Read the model definition and answer for the solid it produces. Units are mm, in the model's axes. Face numbers are marked on the shaded views. A direction names the side the tool comes from. Coordinates: 2 decimals unless noted, no trailing zeros. Loops run counter-clockwise (first coordinate to the right, second up) from the corner with the lowest first, then second, coordinate; pieces in that order, holes last. Notation, with made-up numbers: (5.5, -33.75) -> (25.5, -33.75) arc R14 ccw to (25.5, -25.75) -> close; hole circle Ø2 at (-34.5, 12). An arc over 180 degrees is marked (long way). One line per question, with ' | ' between items. Start each with the question number.
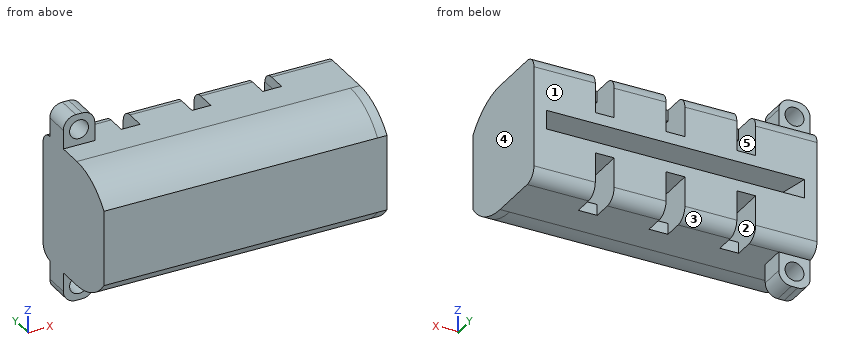
```python
from build123d import *

# Parameters (mm, degrees)
SKETCH1_W            = 90
SKETCH1_H            = 20
BOSS_EXTRUDE1_DEPTH  = 20
SKETCH2_W            = 90
SKETCH2_H            = 3
CUT_EXTRUDE1_DEPTH   = 10
SKETCH3_W            = 3
SKETCH3_H            = 5
CUT_EXTRUDE2_DEPTH   = 10
SKETCH4_W            = 3
SKETCH4_H            = 1.75
SKETCH4_W_2          = 2.997618753
SKETCH4_W_3          = 3.002941468
CUT_EXTRUDE3_DEPTH   = 5
SKETCH5_W            = 1.5
SKETCH5_H            = 3
BOSS_EXTRUDE2_DEPTH  = 10
SKETCH6_W            = 1.5
SKETCH6_H            = 3
BOSS_EXTRUDE3_DEPTH  = 18
BOSS_EXTRUDE4_DEPTH  = 5
FILLET1_START        = 8.5
FILLET1_DEPTH        = 3
FILLET1_START_2      = 8
FILLET1_2_DEPTH      = 4
FILLET2_R            = 10
SKETCH8_W            = 20.140972823
SKETCH8_H            = 2
CUT_EXTRUDE4_DEPTH   = 119
FILLET3_R            = 2
SKETCH9_W            = 5
SKETCH9_H            = 4
BOSS_EXTRUDE6_DEPTH  = 5
SKETCH11_W           = 5
SKETCH11_H           = 4
BOSS_EXTRUDE7_DEPTH  = 5
SKETCH12_R           = 1.5
CUT_EXTRUDE5_DEPTH   = 24
FILLET4_R            = 2
SKETCH14_W           = 71.95999564
SKETCH14_H           = 44.647918029
CUT_EXTRUDE8_DEPTH   = 55
BOSS_EXTRUDE8_START  = 1.5
BOSS_EXTRUDE8_DEPTH  = 1.5
SKETCH16_W           = 5.976122604
SKETCH16_H           = 3
CUT_EXTRUDE9_DEPTH   = 10
SKETCH17_W           = 2
SKETCH17_H           = 3
BOSS_EXTRUDE9_DEPTH  = 10
BOSS_EXTRUDE10_DEPTH = 5


with BuildPart() as part:
    # Sketch1 → Boss-Extrude1 (new body)
    with BuildSketch(Plane.XY):
        with Locations((45, -10)):
            Rectangle(SKETCH1_W, SKETCH1_H)
    extrude(amount=BOSS_EXTRUDE1_DEPTH)

    # Sketch2 → Cut-Extrude1 (cut)
    with BuildSketch(Plane(origin=(0, 0, 0), x_dir=(1, 0, 0), z_dir=(0, 1, 0))):
        with Locations((45, -10)):
            Rectangle(SKETCH2_W, SKETCH2_H)
    extrude(amount=-CUT_EXTRUDE1_DEPTH, mode=Mode.SUBTRACT)

    # Sketch3 → Cut-Extrude2 (cut)
    with BuildSketch(Plane(origin=(0, 0, 0), x_dir=(1, 0, 0), z_dir=(0, 1, 0))):
        with Locations((11.25, -15.75)):
            Rectangle(SKETCH3_W, SKETCH3_H)
        with Locations((22.5, -15.75)):
            Rectangle(SKETCH3_W, SKETCH3_H)
        with Locations((33.75, -15.75)):
            Rectangle(SKETCH3_W, SKETCH3_H)
        with Locations((45, -15.75)):
            Rectangle(SKETCH3_W, SKETCH3_H)
        with Locations((56.25, -15.75)):
            Rectangle(SKETCH3_W, SKETCH3_H)
        with Locations((67.5, -15.75)):
            Rectangle(SKETCH3_W, SKETCH3_H)
        with Locations((78.75, -15.75)):
            Rectangle(SKETCH3_W, SKETCH3_H)
        with Locations((11.25, -4.25)):
            Rectangle(SKETCH3_W, SKETCH3_H)
        with Locations((22.5, -4.25)):
            Rectangle(SKETCH3_W, SKETCH3_H)
        with Locations((33.75, -4.25)):
            Rectangle(SKETCH3_W, SKETCH3_H)
        with Locations((45, -4.25)):
            Rectangle(SKETCH3_W, SKETCH3_H)
        with Locations((56.25, -4.25)):
            Rectangle(SKETCH3_W, SKETCH3_H)
        with Locations((67.5, -4.25)):
            Rectangle(SKETCH3_W, SKETCH3_H)
        with Locations((78.75, -4.25)):
            Rectangle(SKETCH3_W, SKETCH3_H)
    extrude(amount=-CUT_EXTRUDE2_DEPTH, mode=Mode.SUBTRACT)

    # Sketch4 → Cut-Extrude3 (cut)
    with BuildSketch(Plane(origin=(0, 0, 0), x_dir=(1, 0, 0), z_dir=(0, 1, 0))):
        with Locations((56.25, -19.125)):
            Rectangle(SKETCH4_W, SKETCH4_H)
        with Locations((67.5, -19.125)):
            Rectangle(SKETCH4_W, SKETCH4_H)
        Polygon((77.25, -18.25), (77.25, -20), (80.252941468, -20), (80.252941468, -18.25), (80.25, -18.25), align=None)
        with Locations((45, -19.125)):
            Rectangle(SKETCH4_W, SKETCH4_H)
        with Locations((33.748809377, -19.125)):
            Rectangle(SKETCH4_W_2, SKETCH4_H)
        with Locations((22.5, -19.125)):
            Rectangle(SKETCH4_W, SKETCH4_H)
        with Locations((11.25, -19.125)):
            Rectangle(SKETCH4_W, SKETCH4_H)
        with Locations((22.5, -0.875)):
            Rectangle(SKETCH4_W, SKETCH4_H)
        with Locations((33.748809377, -0.875)):
            Rectangle(SKETCH4_W_2, SKETCH4_H)
        with Locations((45, -0.875)):
            Rectangle(SKETCH4_W, SKETCH4_H)
        with Locations((56.25, -0.875)):
            Rectangle(SKETCH4_W, SKETCH4_H)
        with Locations((67.5, -0.875)):
            Rectangle(SKETCH4_W, SKETCH4_H)
        with Locations((78.751470734, -0.875)):
            Rectangle(SKETCH4_W_3, SKETCH4_H)
        with Locations((11.25, -0.875)):
            Rectangle(SKETCH4_W, SKETCH4_H)
    extrude(amount=-CUT_EXTRUDE3_DEPTH, mode=Mode.SUBTRACT)

    # Sketch5 → Boss-Extrude2 (add)
    with BuildSketch(Plane(origin=(0, -10, 0), x_dir=(1, 0, 0), z_dir=(0, 1, 0))):
        with Locations((0.75, -10)):
            Rectangle(SKETCH5_W, SKETCH5_H)
        with Locations((89.25, -10)):
            Rectangle(SKETCH5_W, SKETCH5_H)
    extrude(amount=BOSS_EXTRUDE2_DEPTH)

    # Sketch6 → Boss-Extrude3 (add)
    with BuildSketch(Plane(origin=(0, 0, 0), x_dir=(1, 0, 0), z_dir=(0, 1, 0))):
        with Locations((2.25, -10)):
            Rectangle(SKETCH6_W, SKETCH6_H)
        with Locations((87.75, -10)):
            Rectangle(SKETCH6_W, SKETCH6_H)
    extrude(amount=-BOSS_EXTRUDE3_DEPTH)

    # Sketch7 → Boss-Extrude4 (add)
    with BuildSketch(Plane.XY.offset(8.5)):
        Polygon((3, -9.907661673), (3, -10), (6, -10), (3, 0), align=None)
        Polygon((87, 0), (84, -10), (87, -10), align=None)
    extrude(amount=BOSS_EXTRUDE4_DEPTH)

    # Fillet1: read off the stored shape, not the designer's step
    # Fillet1 outline → Fillet1 (cut)
    with BuildSketch(Plane.XY.offset(FILLET1_START)):
        with BuildLine():
            ThreePointArc((1.511938698, 0), (2.705799758, -0.395414143), (3.427591269, -1.425304229))
            Line((3.427591269, -1.425304229), (3, 0))
            Line((3, 0), (1.511938698, 0))
        make_face()
        with BuildLine():
            Line((87, 0), (86.572408731, -1.425304229))
            ThreePointArc((86.572408731, -1.425304229), (87.294200242, -0.395414143), (88.488061302, 0))
            Line((88.488061302, 0), (87, 0))
        make_face()
    extrude(amount=FILLET1_DEPTH, mode=Mode.SUBTRACT)

    # Fillet1 2 outline → Fillet1 2 (add)
    with BuildSketch(Plane.XY.offset(FILLET1_START_2)):
        with BuildLine():
            Line((6, -10), (7.488061302, -10))
            ThreePointArc((7.488061302, -10), (6.294200242, -9.604585857), (5.572408731, -8.574695771))
            Line((5.572408731, -8.574695771), (6, -10))
        make_face()
        with BuildLine():
            ThreePointArc((84.427591269, -8.574695771), (83.705799758, -9.604585857), (82.511938698, -10))
            Line((82.511938698, -10), (84, -10))
            Line((84, -10), (84.427591269, -8.574695771))
        make_face()
    extrude(amount=FILLET1_2_DEPTH)

    # Fillet2
    fillet2_edges = [part.edges().sort_by_distance(p)[0] for p in [
        (45, -20, 0),
        (45, -20, 20),
    ]]
    fillet(fillet2_edges, radius=FILLET2_R - 0.0001)  # a hair under: the kernel refuses the full size

    # Sketch8 → Cut-Extrude4 (cut)
    with BuildSketch(Plane.ZY):
        with Locations((10.770725067, -19)):
            Rectangle(SKETCH8_W, SKETCH8_H)
    extrude(amount=-CUT_EXTRUDE4_DEPTH, mode=Mode.SUBTRACT)

    # Fillet3
    fillet3_edges = [part.edges().sort_by_distance(p)[0] for p in [
        (4.875, 0, 0),
        (4.875, 0, 20),
        (16.875, 0, 20),
        (16.875, 0, 0),
        (28.125, 0, 0),
        (28.125, 0, 20),
        (39.373809377, 0, 20),
        (39.373809377, 0, 0),
        (50.625, 0, 0),
        (50.625, 0, 20),
        (61.875, 0, 20),
        (61.875, 0, 0),
        (73.125, 0, 0),
        (73.125, 0, 20),
        (85.126470734, 0, 20),
        (85.126470734, 0, 0),
    ]]
    fillet(fillet3_edges, radius=FILLET3_R)

    # Sketch9 → Boss-Extrude6 (add)
    with BuildSketch(Plane.ZY):
        with Locations((-2.5, -4)):
            Rectangle(SKETCH9_W, SKETCH9_H)
        with Locations((22.5, -4)):
            Rectangle(SKETCH9_W, SKETCH9_H)
    extrude(amount=-BOSS_EXTRUDE6_DEPTH)

    # Sketch11 → Boss-Extrude7 (add)
    with BuildSketch(Plane(origin=(90, 0, 0), x_dir=(0, 0, -1), z_dir=(1, 0, 0))):
        with Locations((2.5, -4)):
            Rectangle(SKETCH11_W, SKETCH11_H)
        with Locations((-22.5, -4)):
            Rectangle(SKETCH11_W, SKETCH11_H)
    extrude(amount=-BOSS_EXTRUDE7_DEPTH)

    # Sketch12 → Cut-Extrude5 (cut)
    with BuildSketch(Plane(origin=(0, -2, 0), x_dir=(1, 0, 0), z_dir=(0, 1, 0))):
        with Locations(Location((2.5, 2.5, 0), (0, 0, 180))):
            Circle(SKETCH12_R)
        with Locations(Location((87.5, 2.5, 0), (0, 0, 180))):
            Circle(SKETCH12_R)
        with Locations(Location((87.5, -22.5, 0), (0, 0, 180))):
            Circle(SKETCH12_R)
        with Locations(Location((2.5, -22.5, 0), (0, 0, 180))):
            Circle(SKETCH12_R)
    extrude(amount=-CUT_EXTRUDE5_DEPTH, mode=Mode.SUBTRACT)

    # Fillet4
    fillet4_edges = [part.edges().sort_by_distance(p)[0] for p in [
        (0, -4, -5),
        (5, -4, -5),
        (5, -4, 25),
        (0, -4, 25),
        (85, -4, -5),
        (90, -4, -5),
        (85, -4, 25),
        (90, -4, 25),
    ]]
    fillet(fillet4_edges, radius=FILLET4_R)

    # Sketch14 → Cut-Extrude8 (cut)
    with BuildSketch(Plane(origin=(0, 0, 0), x_dir=(1, 0, 0), z_dir=(0, 1, 0))):
        with Locations((79.47999782, -11.65925291)):
            Rectangle(SKETCH14_W, SKETCH14_H)
    extrude(amount=-CUT_EXTRUDE8_DEPTH, mode=Mode.SUBTRACT)

    # Sketch15 → Boss-Extrude8 (add)
    with BuildSketch(Plane(origin=(43.5, 0, 0), x_dir=(0, 0, -1), z_dir=(1, 0, 0)).offset(BOSS_EXTRUDE8_START)):
        with BuildLine():
            Line((-11.5, 0), (-18, 0))
            ThreePointArc((-18, 0), (-19.414213562, -0.585786438), (-20, -2))
            Line((-20, -2), (-20, -10))
            ThreePointArc((-20, -10), (-18.94427191, -14.472135955), (-16, -18))
            Line((-16, -18), (-4, -18))
            ThreePointArc((-4, -18), (-1.05572809, -14.472135955), (0, -10))
            Line((0, -10), (0, -2))
            ThreePointArc((0, -2), (-0.585786438, -0.585786438), (-2, 0))
            Line((-2, 0), (-4, 0))
            Line((-4, 0), (-8.5, 0))
            Line((-8.5, 0), (-8.5, -10))
            Line((-8.5, -10), (-11.5, -10))
            Line((-11.5, -10), (-11.5, 0))
        make_face()
    extrude(amount=-BOSS_EXTRUDE8_DEPTH)

    # Sketch16 → Cut-Extrude9 (cut)
    with BuildSketch(Plane(origin=(0, 0, 0), x_dir=(1, 0, 0), z_dir=(0, 1, 0))):
        with Locations((4.5, -10)):
            Rectangle(SKETCH16_W, SKETCH16_H)
    extrude(amount=-CUT_EXTRUDE9_DEPTH, mode=Mode.SUBTRACT)

    # Sketch17 → Boss-Extrude9 (add)
    with BuildSketch(Plane(origin=(0, 0, 0), x_dir=(1, 0, 0), z_dir=(0, 1, 0))):
        Polygon((2, -8.5), (1.511938698, -8.5), (0, -8.5), (0, -11.5), (1.511938698, -11.5), (2, -11.5), align=None)
        with Locations((44, -10)):
            Rectangle(SKETCH17_W, SKETCH17_H)
    extrude(amount=-BOSS_EXTRUDE9_DEPTH)

    # Sketch18 → Boss-Extrude10 (add)
    with BuildSketch(Plane.XY.offset(8.5)):
        Polygon((4, -10), (2, 0), (2, -10), align=None)
        Polygon((43, 0), (41, -10), (43, -10), align=None)
    extrude(amount=BOSS_EXTRUDE10_DEPTH)


solid = part.part
```
(1) Section B-B on z = -2.5 is taken. Write down the section's boundary in (x, y).
(2) Find the intervals of material crossed by probe 1 along X at (y, z) = (-7.25, 16); probe 2 along Z at (x, y) = (2.5, -4.4); probe 3 along Z at (x, y) = (31.5, -4.5), in increasing order. Write a range as from..to.
(3) Section D-D on x = 26.5 is taken. Write down the section's boundary in (y, z).
(4) Determine the mould class of the marked faces 1, 2 and 3 for opening direction Z: +Z half, -Z half, draft (parallel to the pull), parting line (faces both ways), or undercut.
(5) Section C-C on y = -7 is taken. Give the number of separate pieces and of enclosed holes in the cut face, plus the area to 3 significant figures.
(6) Each of these flat-tipped pins is pushed along its axis until it touches: pin 1 Ø1.5 at (y, z) = (-4.5, 22) entering from +X; pin 2 Ø2 at (x, y) = (18, -8.5) entering from +Z; pin 3 Ø3.5 at (x, z) = (14.5, 10) entering from +Y; pin 4 Ø2 at (x, y) = (31, -8.5) entering from -Z. Where does it stop, or does it pass through?
(7) A tool of negligible diameter and unlimited length cuts with its end or side. For the marked faces 4 and 5, from which of +Z, -Z, +X, -X, +Y, -Y can it reach the whole face along a straight path? Write none if from no direction.
(8) Section A-A on x = 2.5 is taken. Write down the section's boundary in (y, z).
Working result:
1) outline: (0, -6) -> (1, -6) -> (1, -2) -> (0, -2) -> close; (4, -6) -> (5, -6) -> (5, -2) -> (4, -2) -> close
2) probe 1: x = 0..9.75, 12.75..21, 24..32.25, 35.25..45 | probe 2: z = -5..-4, -1..21, 24..25 | probe 3: z = 0..8.5, 11.5..20
3) outline: (-18, 4) arc R10 ccw to (-10, 0) -> (-2, 0) arc R2 ccw to (0, 2) -> (0, 8.5) -> (-10, 8.5) -> (-10, 11.5) -> (0, 11.5) -> (0, 18) arc R2 ccw to (-2, 20) -> (-10, 20) arc R10 ccw to (-18, 16) -> close
4) face 1: draft | face 2: undercut | face 3: -Z half
5) separate pieces: 1 | enclosed holes: 7 | area: 695 mm2
6) pin 1: stops at x = 5 | pin 2: stops at z = 20 | pin 3: stops at y = 0 | pin 4: stops at z = 0
7) face 4: +Z, -Z, +X, +Y, -Y | face 5: +Y
8) outline: (-18, 4) arc R10 ccw to (-10, 0) -> (-6, 0) -> (-6, -1) -> (-2, -1) -> (-2, 0) arc R2 ccw to (0, 2) -> (0, 8.5) -> (-2.5, 8.5) -> (-2.5, 11.5) -> (0, 11.5) -> (0, 18) arc R2 ccw to (-2, 20) -> (-2, 21) -> (-6, 21) -> (-6, 20) -> (-10, 20) arc R10 ccw to (-18, 16) -> close; (-6, -5) -> (-2, -5) -> (-2, -4) -> (-6, -4) -> close; (-6, 24) -> (-2, 24) -> (-2, 25) -> (-6, 25) -> close
